```python
from build123d import *

# Parameters (mm, degrees)
F1_DEPTH = 10
F3_DEPTH = 25
F4_W     = 42
F4_H     = 2
F5_DEPTH = 20
F6_R     = 2.1
F7_DEPTH = 4
F8_R     = 5
F9_R     = 5


with BuildPart() as f1:
    # F0 (on Top) → F1 (new body)
    with BuildSketch(Plane.XY):
        with BuildLine():
            Line((51.723857, -41.288426), (36.723857, -41.288426))
            ThreePointArc((36.723857, -41.288426), (27.177916, -45.242484), (23.223857, -54.788426))
            Line((23.223857, -54.788426), (23.223857, -64.288426))
            Line((23.223857, -64.288426), (65.223857, -64.288426))
            Line((65.223857, -64.288426), (65.223857, -54.788426))
            ThreePointArc((65.223857, -54.788426), (61.269799, -45.242484), (51.723857, -41.288426))
        make_face()
    extrude(amount=F1_DEPTH)

    # F2 (on face) → F3 (cut)
    with BuildSketch(Plane.XY.offset(10)):
        with BuildLine():
            Line((51.723857, -43.288426), (36.723857, -43.288426))
            ThreePointArc((36.723857, -43.288426), (28.592129, -46.656698), (25.223857, -54.788426))
            Line((25.223857, -54.788426), (25.223857, -62.288426))
            Line((25.223857, -62.288426), (63.223857, -62.288426))
            Line((63.223857, -62.288426), (63.223857, -54.788426))
            ThreePointArc((63.223857, -54.788426), (59.855585, -46.656698), (51.723857, -43.288426))
        make_face()
    extrude(amount=-F3_DEPTH, mode=Mode.SUBTRACT)

    # F4 (on face) → F5 (join)
    with BuildSketch(Plane.XY.offset(10)):
        with Locations((44.223857, -63.288426)):
            Rectangle(F4_W, F4_H)
    extrude(amount=F5_DEPTH)

    # F6 (on face) → F7 (cut)
    with BuildSketch(Plane.XZ.offset(64.288426)):
        with Locations((44.223857, 20)):
            Circle(F6_R)
    extrude(amount=-F7_DEPTH, mode=Mode.SUBTRACT)

    # F8
    f8_edges = [f1.edges().sort_by_distance(p)[0] for p in [
        (65.223857, -63.288426, 30),
    ]]
    fillet(f8_edges, radius=F8_R)

    # F9
    f9_edges = [f1.edges().sort_by_distance(p)[0] for p in [
        (23.223857, -63.288426, 30),
    ]]
    fillet(f9_edges, radius=F9_R)


solid = f1.part
```
Here's how the part is built. I have some questions about the finished solid (model axes, mm). A direction names the side the tool comes from. Give positions to 0.01 mm unless a question says otherwise; leave off trailing zeros. Order: outer loops, then holes, each group sorted by start corner. A loop starts at its lowest first (then second) coordinate and runs counter-clockwise, first axis right, second up. Notation, with made-up numbers: M -17.5,-26 L 1.5,-26 A23 cw 1.5,-7 Z; hole C 11,76.5 d1. An arc over 180 degrees is marked long. Use a Markdown table: item, result. Add a question column.
1. Suppose I cut it at B-B (z = 20). List the corners of the cut face in (x, y) for me, and give its area (3 significant figures).
2. For pin 1 Ø6.5 at (x, z) = (44.22, 20) entering from +Y; pin 2 Ø3 at (y, z) = (-51.5, 9) entering from +X; pin 3 Ø12 at (x, z) = (58.5, 7) entering from +Y, each with a flat end and sliding along its axis, tell me the tip position at first contact or that it passes through.
3. If we mould it in two halves opening along Z, with no side actions, what happens to faces 4 (the cylindrical face through (28.68, -46.57, 5.07)), 5 (the cylindrical face through (45.353, -63.302, 21.771)), 6 (the cylindrical face through (63.72, -63.274, 28.574))? For each: +Z half, -Z half, draft (parallel to the pull), parting line (faces both ways), or undercut.
4. I need wall thicknesses on probe 1 along X at (y, z) = (-58.5, 8.75); probe 2 along Y at (x, z) = (46, 9.25); probe 3 along Y at (x, z) = (26.5, 16). Which ranges of each line are inside material? Lowest first, please. Write a range as from..to.
5. Suppose I cut it at C-C (z = 6). List the corners of the cut face in (x, y) for me, and give its area (3 significant figures).
6. Suppose I cut it at A-A (y = -56.25). List the corners of the cut face in (x, z) for me.
7. On a 3-axis mill with a long thin cutter (end or side, diameter ignored), from which of +Z, -Z, +X, -X, +Y, -Y can I reach the whole of each face in a straight line? I mean faces 1 (the flat face through (44, -43, 10)), 2 (the flat face through (44, -63, 0)), 3 (the flat face through (44, -43.288, 5)). Say none if no direction works.
Results list:
| question | item | result |
|---|---|---|
| 1 | outline | M 23.22,-64.29 L 42.12,-64.29 L 42.12,-62.29 L 23.22,-62.29 Z; M 46.32,-64.29 L 65.22,-64.29 L 65.22,-62.29 L 46.32,-62.29 Z |
| 1 | area | 75.6 mm² |
| 2 | pin 1 | stops at y = -62.29 |
| 2 | pin 2 | stops at x = 65.1 |
| 2 | pin 3 | stops at y = -41.31 |
| 3 | face 4 | draft |
| 3 | face 5 | undercut |
| 3 | face 6 | +Z half |
| 4 | probe 1 | x = 23.22..25.22, 63.22..65.22 |
| 4 | probe 2 | y = -64.29..-62.29, -43.29..-41.29 |
| 4 | probe 3 | y = -64.29..-62.29 |
| 5 | outline | M 23.22,-64.29 L 65.22,-64.29 L 65.22,-54.79 A13.5 ccw 51.72,-41.29 L 36.72,-41.29 A13.5 ccw 23.22,-54.79 Z; hole M 25.22,-62.29 L 63.22,-62.29 L 63.22,-54.79 A11.5 ccw 51.72,-43.29 L 36.72,-43.29 A11.5 ccw 25.22,-54.79 Z |
| 5 | area | 223 mm² |
| 6 | outline | M 23.22,0 L 25.22,0 L 25.22,10 L 23.22,10 Z; M 63.22,0 L 65.22,0 L 65.22,10 L 63.22,10 Z |
| 7 | face 1 | +Z, +X, -X, +Y |
| 7 | face 2 | -Z, +X, -X, +Y, -Y |
| 7 | face 3 | +Z, -Z |
